from build123d import *

# Parameters (mm, degrees)
BASE_FLANGE1_DEPTH      = 0.7
EDGE_FLANGE1_DEPTH      = 17.5
EDGE_FLANGE1_BEND_DEPTH = 37.5
BREAK_CORNER1_START     = -1.7
BREAK_CORNER1_DEPTH     = 0.7
BREAK_CORNER1_2_DEPTH   = 0.7
BREAK_CORNER1_START_2   = -0.7
BREAK_CORNER1_3_DEPTH   = 0.7


# Read off the part's stored shape, not the designer's step: Break-Corner1
# Sheet-metal steps are written as plain solids
with BuildPart() as part:
    # Sketch1 → Base-Flange1 (new body)
    with BuildSketch(Plane(origin=(0, 0, 0), x_dir=(1, 0, 0), z_dir=(0, 1, 0))):
        Polygon((0, 0), (0, -20), (39.39231012, 6.945927107), align=None)
    extrude(amount=-BASE_FLANGE1_DEPTH)

    # Edge-Flange1 section (across the edge) → Edge-Flange1 (add)
    with BuildSketch(Plane(origin=(-1, 0, 2.5), x_dir=(1, 0, 0), z_dir=(0, 0, 1))):
        with BuildLine():
            Line((-0.7, 1), (-0.7, 10))
            Line((-0.7, 10), (0, 10))
            Line((0, 10), (0, 1))
            ThreePointArc((0, 1), (0.292893219, 0.292893219), (1, 0))
            Line((1, 0), (1, -0.7))
            ThreePointArc((1, -0.7), (-0.202081528, -0.202081528), (-0.7, 1))
        make_face()
    extrude(amount=EDGE_FLANGE1_DEPTH)

    # Edge-Flange1 section 2 (across the edge) → Edge-Flange1 bend (add)
    with BuildSketch(Plane(origin=(39.218661943, 0, -7.93073486), x_dir=(0.1736481776669273, 3.4914813388431334e-15, 0.9848077530122086), z_dir=(-0.9848077530122086, 0, 0.1736481776669273))):
        with BuildLine():
            Line((-0.7, 1), (-0.7, 10))
            Line((-0.7, 10), (0, 10))
            Line((0, 10), (0, 1))
            ThreePointArc((0, 1), (0.292893219, 0.292893219), (1, 0))
            Line((1, 0), (1, -0.7))
            ThreePointArc((1, -0.7), (-0.202081528, -0.202081528), (-0.7, 1))
        make_face()
    extrude(amount=EDGE_FLANGE1_BEND_DEPTH)

    # Break-Corner1 outline → Break-Corner1 (cut)
    with BuildSketch(Plane(origin=(0, 0, 0), x_dir=(0.9848077530122086, 0, -0.173648177666927), z_dir=(0.17364817766692697, 0, 0.9848077530122088)).offset(BREAK_CORNER1_START)):
        with BuildLine():
            ThreePointArc((2.5, 7.5), (3.232233047, 9.267766953), (5, 10))
            Line((5, 10), (2.5, 10))
            Line((2.5, 10), (2.5, 7.5))
        make_face()
        with BuildLine():
            ThreePointArc((37.5, 10), (39.267766953, 9.267766953), (40, 7.5))
            Line((40, 7.5), (40, 10))
            Line((40, 10), (37.5, 10))
        make_face()
    extrude(amount=BREAK_CORNER1_DEPTH, mode=Mode.SUBTRACT)

    # Break-Corner1 2 outline → Break-Corner1 2 (cut)
    with BuildSketch(Plane.YZ.offset(BREAK_CORNER1_START)):
        with BuildLine():
            ThreePointArc((7.5, 20), (9.267766953, 19.267766953), (10, 17.5))
            Line((10, 17.5), (10, 20))
            Line((10, 20), (7.5, 20))
        make_face()
        with BuildLine():
            ThreePointArc((10, 5), (9.267766953, 3.232233047), (7.5, 2.5))
            Line((7.5, 2.5), (10, 2.5))
            Line((10, 2.5), (10, 5))
        make_face()
    extrude(amount=BREAK_CORNER1_2_DEPTH, mode=Mode.SUBTRACT)

    # Break-Corner1 3 outline → Break-Corner1 3 (cut)
    with BuildSketch(Plane(origin=(0, 0, 0), x_dir=(1, 0, 0), z_dir=(0, 1, 0)).offset(BREAK_CORNER1_START_2)):
        with BuildLine():
            ThreePointArc((0, -2.097749078), (0.584888892, -0.490780054), (2.065879556, 0.364270305))
            Line((2.065879556, 0.364270305), (0, 0))
            Line((0, 0), (0, -2.097749078))
        make_face()
    extrude(amount=BREAK_CORNER1_3_DEPTH, mode=Mode.SUBTRACT)


solid = part.part
CAD build for the part. Positions are in the model's coordinates, mm. A direction names the side the tool comes from. Give positions to 0.01 mm unless a question says otherwise; leave off trailing zeros. Write each loop counter-clockwise with the first axis right and the second up, starting at its lowest first coordinate (ties: lowest second). Pieces come first, ordered by that corner, then holes. Notation, with made-up numbers: (49.25, 12.5) - (94.25, 12.5) arc R18 ccw to (94.25, 44.5) - close; hole circle Ø8 at (34.25, -39.75). An arc over 180 degrees is marked (long way). Put each result on its own line as item: value.
(1) Saw through at B-B (z = 6.5). List the corners of the cut face in (x, y).
Working result:
outline: (-1.7, 1) arc R1.7 ccw to (0, -0.7) - (19.74, -0.7) - (19.74, 0) - (0, 0) arc R1 cw to (-1, 1) - (-1, 10) - (-1.7, 10) - close
(2) Saw through at A-A (y = 6.75). List the corners of the cut face in (x, z).
Working result:
outline: (-1.7, 2.5) - (-1, 2.5) - (-1, 20) - (-1.7, 20) - close; (2.17, -2.11) - (39.1, -8.62) - (39.22, -7.93) - (2.29, -1.42) - close
(3) Wall check: L1, parallel to Y at x = 11, z = 11.25; L2, parallel to X at y = 6.75, z = 15.5; L3, parallel to Z at x = 28, y = 6.25. Give the ranges that are in metal, low to high.
Working result:
L1: -0.7 to 0
L2: -1.7 to -1
L3: -6.66 to -5.95
(4) Pull direction Z, two halves, no side cores. Call faces 1 (the flat face through (2.25, 3.46, -1.63)), 2 (the flat face through (20.89, 5.44, -5.41)), 3 (the flat face through (-1, 6, 11)): released by +Z, released by -Z, zero draft, split by the parting line, or undercut.
Working result:
face 1: undercut
face 2: released by -Z
face 3: zero draft
(5) Saw through at C-C (z = 14). List the corners of the cut face in (x, y), then the cut area to 3 significant figures.
Working result:
outline: (-1.7, 1) arc R1.7 ccw to (0, -0.7) - (8.77, -0.7) - (8.77, 0) - (0, 0) arc R1 cw to (-1, 1) - (-1, 10) - (-1.7, 10) - close
area: 13.9 mm^2
(6) Tool access for faces 4 (the flat face through (-1.2, 3.5, 2.5)), 5 (the cylindrical face through (-0.715, 0.301, 11.128)), 6 (the flat face through (21.01, 5.56, -4.72)): list every direction of +Z, -Z, +X, -X, +Y, -Y with a clear straight run to the whole face (end or side of a thin tool).
Working result:
face 4: -Z, -X, +Y, -Y
face 5: +Z, -Z, +X, +Y
face 6: +Z, +X, +Y
(7) Drop flat-ended pins along their axis: pin 1 Ø4 at (y, z) = (3, 14.5) entering from +X; pin 2 Ø1.5 at (x, y) = (17, 6) entering from +Z; pin 3 Ø5 at (x, y) = (15, 9) entering from -Z. Give the stop position or say it passes through.
Working result:
pin 1: x = -1
pin 2: z = -3.88
pin 3: z = -4.81
